Model file for the job. Use its own axes, mm. Round coordinates to 2 decimals unless told otherwise and drop trailing zeros. Order: outer loops, then holes, each group sorted by start corner. A loop starts at its lowest first (then second) coordinate and runs counter-clockwise, first axis right, second up. Notation, with made-up numbers: (-32, 0) - (5, 0) arc R25 ccw to (5, 25) - close; hole circle Ø11 at (-10, -19.5). An arc over 180 degrees is marked (long way). Write item = value, one per line.
```python
from build123d import *

# Parameters (mm, degrees)
SKETCH_W  = 120
SKETCH_H  = 120
PAD_DEPTH = 10
FILLET_R  = 9


with BuildPart() as part:
    # Sketch → Pad (new body)
    with BuildSketch(Plane.XZ):
        Rectangle(SKETCH_W, SKETCH_H)
    extrude(amount=PAD_DEPTH)

    # Fillet
    fillet_edges = [part.edges().sort_by_distance(p)[0] for p in [
        (-60, -5, 60),
        (0, 0, 60),
        (-60, 0, 0),
        (60, -5, 60),
        (60, 0, 0),
        (60, -5, -60),
        (0, 0, -60),
        (-60, -5, -60),
    ]]
    fillet(fillet_edges, radius=FILLET_R)


solid = part.part
```
1) Cut at C-C (x = 21). Write the cut outline in (y, z), and give its area (3 significant figures).
Conclusion:
outline = (-10, -60) - (-9, -60) arc R9 ccw to (0, -51) - (0, 51) arc R9 ccw to (-9, 60) - (-10, 60) - close
area = 1,170 mm^2
2) Cut at A-A (y = -6.5). Write the cut outline in (x, z), and give its area (3 significant figures).
Conclusion:
outline = (-59.65, -51) arc R8.65 ccw to (-51, -59.65) - (51, -59.65) arc R8.65 ccw to (59.65, -51) - (59.65, 51) arc R8.65 ccw to (51, 59.65) - (-51, 59.65) arc R8.65 ccw to (-59.65, 51) - close
area = 14,200 mm^2
3) Cut at B-B (z = -41). Write the cut outline in (x, y).
Conclusion:
outline = (-60, -10) - (60, -10) - (60, -9) arc R9 ccw to (51, 0) - (-51, 0) arc R9 ccw to (-60, -9) - close
4) Wall check: line 1 along Z through (x, y) = (-4, -8.25); line 2 along Z through (x, y) = (-53, -2); line 3 along X through (y, z) = (-2.75, 53). Give the ranges that are in metal, low to high.
Conclusion:
line_1 = -59.97 to 59.97
line_2 = -56.29 to 56.29
line_3 = -57.16 to 57.16
5) Flat gauge pins, fed straight in: pin 1 Ø3 at (x, y) = (-11.5, -3.5) entering from -Z; pin 2 Ø5 at (x, y) = (2, -3.5) entering from +Z; pin 3 Ø3 at (x, y) = (31, -2.5) entering from -Z. Where does each tip first touch, or does it go through?
Conclusion:
pin_1 = -59.06
pin_2 = 59.49
pin_3 = -58.48
